Geometry check sheet. Reference: the model listing, model coordinates, mm. A direction names the side the tool comes from. Round coordinates to 2 decimals unless told otherwise and drop trailing zeros. Loops run counter-clockwise (first coordinate to the right, second up) from the corner with the lowest first, then second, coordinate; pieces in that order, holes last. Notation, with made-up numbers: (3.25, 81.5) - (40.25, 81.5) arc R25 ccw to (40.25, 116.5) - close; hole circle Ø5 at (48, 54.25). An arc over 180 degrees is marked (long way). Answer as CSV lines item,"result". Start each with the question number.
1) Access from +Z, -Z, +X, -X, +Y, -Y to the whole of each face (thin tool, end or side, straight path). Record for faces 4 (the cylindrical face through (27.23, 3.22, 7.79)), 5 (the flat face through (0, 0, 0)).
2) Depth check by flat-ended pin: P1, Ø0.8, axis at x = -27.5, z = 7.5, coming from the +Y side; P2, Ø6, axis at x = 0.5, z = 7, coming from the +Y side; P3, Ø1.6, axis at x = 27, z = 7.5, coming from the +Y side. Enter the tip coordinate at first touch or a pass-through.
3) Cross-section at B-B on y = 8.5. Record the boundary of the cut face in (x, z), and give its area (3 significant figures).
4) Cross-section at A-A on z = -5.25. Record the boundary of the cut face in (x, y).
5) Thickness scan on line 1 along Z through (x, y) = (27, 9.25); line 2 along Z through (x, y) = (20.5, 2.5); line 3 along X through (y, z) = (3.5, -8.25). Record the ranges inside material, lowest first.
6) Cross-section at D-D on x = -23.5. Record the boundary of the cut face in (y, z), and give its area (3 significant figures).
7) Cross-section at C-C on x = 24. Record the boundary of the cut face in (y, z).
8) Draft check along X on faces 1 (the flat face through (21, 5.5, 8)), 2 (the flat face through (-27, 3, -6.25)), 3 (the flat face through (30, 6, 0)). Enter one of: released by +X, released by -X, zero draft, split by the parting line, or undercut.
from build123d import *

# Parameters (mm, degrees)
SKETCH1_W           = 60
SKETCH1_H           = 20
BOSS_EXTRUDE1_DEPTH = 9.5
SHELL1_T            = -1
SKETCH2_W           = 12.5
SKETCH2_H           = 4.7
CUT_EXTRUDE1_DEPTH  = 12
SKETCH3_W           = 19.267308131
SKETCH3_H           = 2.75
SKETCH3_R           = 0.75
SKETCH3_W_2         = 2.75
BOSS_EXTRUDE2_DEPTH = 4.5
FILLET1_R           = 5
FILLET2_R           = 5


with BuildPart() as part:
    # Sketch1 → Boss-Extrude1 (new body)
    with BuildSketch(Plane(origin=(0, 0, 0), x_dir=(1, 0, 0), z_dir=(0, 1, 0))):
        Rectangle(SKETCH1_W, SKETCH1_H)
    extrude(amount=BOSS_EXTRUDE1_DEPTH)

    # Shell1
    shell1_openings = [part.faces().sort_by_distance(p)[0] for p in [
        (0, 9.5, 0),
    ]]
    offset(amount=SHELL1_T, openings=shell1_openings, kind=Kind.INTERSECTION)

    # Sketch2 → Cut-Extrude1 (cut)
    with BuildSketch(Plane(origin=(30, 0, 0), x_dir=(0, 0, -1), z_dir=(1, 0, 0))):
        with Locations((0, 3.35)):
            Rectangle(SKETCH2_W, SKETCH2_H)
    extrude(amount=-CUT_EXTRUDE1_DEPTH, mode=Mode.SUBTRACT)

    # Sketch3 → Boss-Extrude2 (add)
    # profile 1 of 4: a face of its own
    with BuildSketch(Plane(origin=(0, 1, 0), x_dir=(1, 0, 0), z_dir=(0, 1, 0))):
        with Locations((19.366345935, 7.625)):
            Rectangle(SKETCH3_W, SKETCH3_H)
        with Locations(Location((26.5, 7.625, 0), (0, 0, 270))):
            Circle(SKETCH3_R, mode=Mode.SUBTRACT)
    # profile 2 of 4: a face of its own
    with BuildSketch(Plane(origin=(0, 1, 0), x_dir=(1, 0, 0), z_dir=(0, 1, 0))):
        with Locations((-27.625, 7.625)):
            Rectangle(SKETCH3_W_2, SKETCH3_H)
        with Locations(Location((-27.625, 7.625, 0), (0, 0, 270))):
            Circle(SKETCH3_R, mode=Mode.SUBTRACT)
    # profile 3 of 4: a face of its own
    with BuildSketch(Plane(origin=(0, 1, 0), x_dir=(1, 0, 0), z_dir=(0, 1, 0))):
        with Locations((-27.625, -7.625)):
            Rectangle(SKETCH3_W_2, SKETCH3_H)
        with Locations(Location((-27.625, -7.625, 0), (0, 0, 90))):
            Circle(SKETCH3_R, mode=Mode.SUBTRACT)
    # profile 4 of 4: a face of its own
    with BuildSketch(Plane(origin=(0, 1, 0), x_dir=(1, 0, 0), z_dir=(0, 1, 0))):
        with Locations((19.366345935, -7.625)):
            Rectangle(SKETCH3_W, SKETCH3_H)
        with Locations(Location((26.5, -7.625, 0), (0, 0, 90))):
            Circle(SKETCH3_R, mode=Mode.SUBTRACT)
    extrude(amount=BOSS_EXTRUDE2_DEPTH)

    # Fillet1
    # the kernel refuses this fillet: 5 mm, written as the material it adds along each edge
    with BuildSketch(Plane(origin=(-26.25, 1, 9), x_dir=(1, 0, 0), z_dir=(0, 0, -1))) as fillet1_piece_1:
        with BuildLine():
            CenterArc((4.974937186, -5), FILLET1_R, 90, 84.260829523)
            Line((0, -4.5), (-0.099498744, -4.49))
            ThreePointArc((-0.099498744, -4.49), (-0.1, -2.25), (-0.1, 0))
            Line((-0.1, 0), (0, 0.1))
            Line((0, 0.1), (4.974937186, 0.1))
            Line((4.974937186, 0.1), (4.974937186, 0))
        make_face()
    extrude(amount=2.75)
    with BuildSketch(Plane(origin=(-26.25, 1, -9), x_dir=(1, 0, 0), z_dir=(0, 0, 1)), Plane(origin=(9.732691869, 1, 9), x_dir=(-1, 0, 0), z_dir=(0, 0, -1))) as fillet1_piece_2:
        with BuildLine():
            CenterArc((4.974937186, 5), FILLET1_R, 185.739170477, 84.260829523)
            Line((0, 4.5), (-0.099498744, 4.49))
            ThreePointArc((-0.099498744, 4.49), (-0.1, 2.25), (-0.1, 0))
            Line((-0.1, 0), (0, -0.1))
            Line((0, -0.1), (4.974937186, -0.1))
            Line((4.974937186, -0.1), (4.974937186, 0))
        make_face()
    extrude(amount=2.75)
    with BuildSketch(Plane(origin=(9.732691869, 1, -9), x_dir=(0, 1, 0), z_dir=(0, 0, 1))) as fillet1_piece_3:
        with BuildLine():
            CenterArc((5, 4.974937186), FILLET1_R, 180, 84.260829523)
            Line((0, 4.974937186), (-0.1, 4.974937186))
            Line((-0.1, 4.974937186), (-0.1, 0))
            Line((-0.1, 0), (0, -0.1))
            ThreePointArc((0, -0.1), (2.25, -0.1), (4.49, -0.099498744))
            Line((4.49, -0.099498744), (4.5, 0))
        make_face()
    extrude(amount=2.75)

    # Fillet2
    fillet2_edges = [part.edges().sort_by_distance(p)[0] for p in [
        (9.732691869, 5.5, -7.625),
        (9.732691869, 5.5, 7.625),
    ]]
    fillet(fillet2_edges, radius=FILLET2_R)


solid = part.part
Answer block:
1,face 4,"+Y"
1,face 5,"+Z, -Z, +X, -X, -Y"
2,P1,"stops at y = 1"
2,P2,"stops at y = 9.5"
2,P3,"stops at y = 5.5"
3,outline,"(-30, -10) - (30, -10) - (30, 10) - (-30, 10) - close; hole (-29, -9) - (29, -9) - (29, 9) - (-29, 9) - close"
3,area,"156 mm^2"
4,outline,"(-30, 0) - (30, 0) - (30, 1) - (-29, 1) - (-29, 9.5) - (-30, 9.5) - close; (29, 5.7) - (30, 5.7) - (30, 9.5) - (29, 9.5) - close"
5,line 1,"z = -10 to -9, 9 to 10"
5,line 2,"z = -10 to -6.25, 6.25 to 10"
5,line 3,"x = -30 to -28.04, -27.21 to -25.61, 9.11 to 26.09, 26.91 to 30"
6,outline,"(0, -10) - (9.5, -10) - (9.5, -9) - (1.52, -9) - (1.52, -6.25) - (1, -6.25) - (1, 6.25) - (1.52, 6.25) - (1.52, 9) - (9.5, 9) - (9.5, 10) - (0, 10) - close"
6,area,"39.9 mm^2"
7,outline,"(0, -10) - (9.5, -10) - (9.5, -9) - (5.5, -9) - (5.5, -6.25) - (1, -6.25) - (1, 6.25) - (5.5, 6.25) - (5.5, 9) - (9.5, 9) - (9.5, 10) - (0, 10) - close"
8,face 1,"undercut"
8,face 2,"zero draft"
8,face 3,"released by +X"
